Input: part model. Units: mm. Frame: model coordinates. Coordinates: 2 decimals unless noted, no trailing zeros. Write each loop counter-clockwise with the first axis right and the second up, starting at its lowest first coordinate (ties: lowest second). Pieces come first, ordered by that corner, then holes. Notation, with made-up numbers: (16, -10) -> (28, -10) arc R18 ccw to (28, 23) -> close; hole circle Ø2 at (-30.75, 36). An arc over 180 degrees is marked (long way). Use one line per item in the form item = value. Start each with the question number.
(1) Cut plane D-D on x = -5.5. Return the cut outline in (y, z).
(2) Cut plane A-A on y = -3. Return the cut outline in (x, z), plus the area to 3 significant figures.
(3) Ray query, line 1 along Y through (x, z) = (-41, 1.95); line 2 along Y through (x, z) = (-0.5, 1); line 3 along Y through (x, z) = (-22, 1.35). Return the intervals inside material, ascending.
(4) Cut plane C-C on z = 1.9. State how many separate pieces and enclosed holes the cut face has, plus the area to 3 significant figures.
(5) First-contact query: pin 1 (2 mm diameter, centred on x = -3.5, z = 1.5, fed in from +Y); pin 2 (7 mm diameter, centred on x = -41, y = 10, fed in from -Z). Flat tips, straight axial feed; report the tip coordinate or a pass-through.
(6) Cut plane B-B on x = -41. Return the cut outline in (y, z), plus the area to 3 significant figures.
Autodesk Inventor part; units mm, degrees
ref_plane "YZ Plane" through (0, 0, 0) normal (1, 0, 0) x (0, 1, 0)
ref_plane "XZ Plane" through (0, 0, 0) normal (0, 1, 0) x (-1, 0, 0)
ref_plane "XY Plane" through (0, 0, 0) normal (0, 0, 1) x (1, 0, 0)
sketch "Эскиз1" plane through (0, 0, 0) normal (0, 0, 1) x (1, 0, 0)
  circle A0 centre (-41, -10) radius 4
  circle A1 centre (-41, 10) radius 4
  circle A2 centre (41, 10) radius 4
  circle A3 centre (41, -10) radius 4
  line L0 (-41, 10) -> (41, 10) construction
  line L1 (41, 10) -> (41, -10) construction
  line L2 (41, -10) -> (-41, -10) construction
  line L3 (-41, -10) -> (-41, 10) construction
  arc A4 (-33, 10) -> (-49, 10) centre (-41, 10) ccw
  arc A5 (-49, -10) -> (-33, -10) centre (-41, -10) ccw
  arc A6 (33, -10) -> (49, -10) centre (41, -10) ccw
  arc A7 (49, 10) -> (33, 10) centre (41, 10) ccw
  line L4 (-49, 10) -> (-49, -10)
  line L5 (49, 10) -> (49, -10)
  line L6 (33, 10) -> (-33, 10)
  line L7 (33, -10) -> (-33, -10)
  line L8 (13, -2) -> (-13, -2)
  line L9 (-13, -2) -> (-13, 2)
  line L10 (-13, 2) -> (13, 2)
  line L11 (13, 2) -> (13, -2)
  line L12 (-24, 5) -> (-20, 5)
  line L13 (-20, 5) -> (-20, -5)
  line L14 (-20, -5) -> (-24, -5)
  line L15 (-24, -5) -> (-24, 5)
  line L16 (20, -5) -> (24, -5)
  line L17 (24, -5) -> (24, 5)
  line L18 (24, 5) -> (20, 5)
  line L19 (20, 5) -> (20, -5)
  line L20 (0, -10) -> (0, 10)
  point P0 (0, 0)
  point P1 (41, 0)
  point P2 (0, 2)
  point P3 (13, 0)
  point P4 (-20, 0)
  point P5 (-13, 0)
  dimension "d0" = 8
  dimension "d1" = 20
  dimension "d2" = 82
  dimension "d3" = 8
  dimension "d6" = 10
  dimension "d7" = 10
  dimension "d8" = 4
  dimension "d9" = 26
  dimension "d10" = 10
  dimension "d11" = 40
extrude "Выдавливание1" add sketch "Эскиз1" along normal blind 4 contours L6 L20 L10 L9 L8 L7 A5 L4 A4 | L6 A7 L5 A6 L7 L20 L8 L11 L10
sketch "Эскиз2" plane through (0, 0, 4) normal (0, 0, 1) x (1, 0, 0)
  line L0 (-13, -2) -> (-13, 2)
  line L1 (-13, 2) -> (13, 2)
  line L2 (13, 2) -> (13, -2)
  line L3 (13, -2) -> (-13, -2)
  circle A0 centre (41, -10) radius 4
  circle A1 centre (41, 10) radius 4
  circle A2 centre (-41, 10) radius 4
  circle A3 centre (-41, -10) radius 4
  line L4 (20, -5) -> (20, 5)
  line L5 (20, 5) -> (24, 5)
  line L6 (24, 5) -> (24, -5)
  line L7 (24, -5) -> (20, -5)
  line L8 (-20, 5) -> (-20, -5)
  line L9 (-20, -5) -> (-24, -5)
  line L10 (-24, -5) -> (-24, 5)
  line L11 (-24, 5) -> (-20, 5)
  arc A4 (-33, 10) -> (-49, 10) centre (-41, 10) ccw
  line L12 (-49, 10) -> (-49, -10)
  arc A5 (-49, -10) -> (-33, -10) centre (-41, -10) ccw
  line L13 (-33, -10) -> (33, -10)
  arc A6 (33, -10) -> (49, -10) centre (41, -10) ccw
  line L14 (49, -10) -> (49, 10)
  arc A7 (49, 10) -> (33, 10) centre (41, 10) ccw
  line L15 (33, 10) -> (-33, 10)
  point P0 (0, 0)
  point P1 (-41, 0)
  point P2 (41, 0)
hole "Отверстие1" at (-41, 0, 4) at (41, 0, 4) direction (0, 0, -1) diameter 3 end through all
properties part number "PistonPart1" material "Дерево (вишня)"
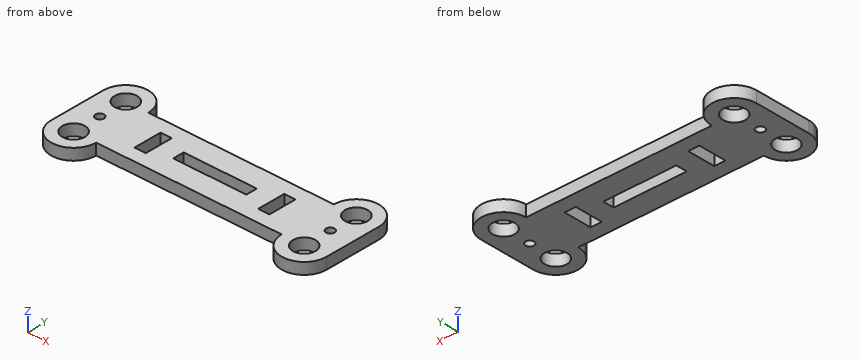
Values:
q1.outline = (-10, 0) -> (-2, 0) -> (-2, 4) -> (-10, 4) -> close; (2, 0) -> (10, 0) -> (10, 4) -> (2, 4) -> close
q2.outline = (-49, 0) -> (-24, 0) -> (-24, 4) -> (-49, 4) -> close; (-20, 0) -> (20, 0) -> (20, 4) -> (-20, 4) -> close; (24, 0) -> (49, 0) -> (49, 4) -> (24, 4) -> close
q2.area = 360 mm2
q3.line_1 = -18 to -14, -6 to -1.5, 1.5 to 6, 14 to 18
q3.line_2 = -10 to -2, 2 to 10
q3.line_3 = -10 to -5, 5 to 10
q4.separate_pieces = 1
q4.enclosed_holes = 9
q4.area = 1,960 mm2
q5.pin_1 = 10
q5.pin_2 = through
q6.outline = (-18, 0) -> (-14, 0) -> (-14, 4) -> (-18, 4) -> close; (-6, 0) -> (-1.5, 0) -> (-1.5, 4) -> (-6, 4) -> close; (1.5, 0) -> (6, 0) -> (6, 4) -> (1.5, 4) -> close; (14, 0) -> (18, 0) -> (18, 4) -> (14, 4) -> close
q6.area = 68.0 mm2
